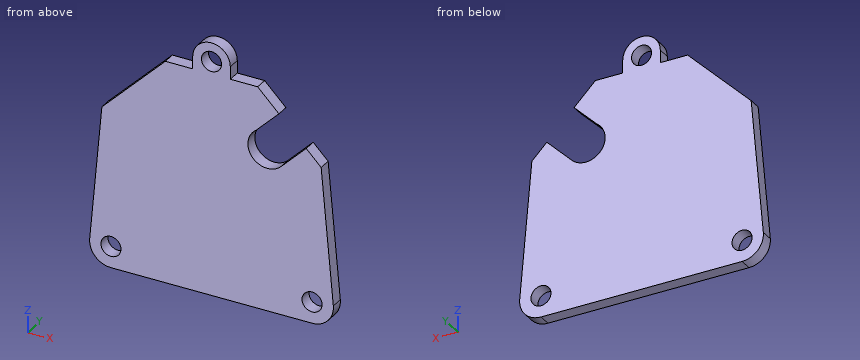
```python
from build123d import *

# Parameters (mm, degrees)
SKETCH1_R           = 1.6
BOSS_EXTRUDE1_DEPTH = 2


with BuildPart() as part:
    # Sketch1 → Boss-Extrude1 (new body)
    with BuildSketch(Plane(origin=(0, 0, 0), x_dir=(1, 0, 0), z_dir=(0, 1, 0))):
        with BuildLine():
            ThreePointArc((7.536585866, 10.5201286), (2.958706846, 10.319962474), (3.565513998, 5.778065527))
            Line((3.565513998, 5.778065527), (7.192643667, 2.150935858))
            Line((7.192643667, 2.150935858), (3.793373086, -1.248334723))
            Line((3.793373086, -1.248334723), (-0.570702654, -1.248334723))
            Line((-0.570702654, -1.248334723), (-0.570702654, -3.253047476))
            ThreePointArc((-0.570702654, -3.253047476), (-3.570702654, -6.253047476), (-6.570702654, -3.253047476))
            Line((-6.570702654, -3.253047476), (-6.570702654, -1.248334723))
            Line((-6.570702654, -1.248334723), (-10.934778393, -1.248334723))
            Line((-10.934778393, -1.248334723), (-21.070702654, 8.887589537))
            Line((-21.070702654, 8.887589537), (-23.015874855, 30.595563989))
            ThreePointArc((-23.015874855, 30.595563989), (-22.136333563, 33.200086558), (-19.620702654, 34.308568326))
            Line((-19.620702654, 34.308568326), (12.479297346, 34.308568326))
            ThreePointArc((12.479297346, 34.308568326), (14.994928256, 33.200086558), (15.874469548, 30.595563989))
            Line((15.874469548, 30.595563989), (13.929297346, 8.887589537))
            Line((13.929297346, 8.887589537), (11.545749837, 6.504042028))
            Line((11.545749837, 6.504042028), (7.536585866, 10.5201286))
        make_face()
        with Locations((-19.620702654, 30.899792953)):
            Circle(SKETCH1_R, mode=Mode.SUBTRACT)
        with Locations((12.479297346, 30.899792953)):
            Circle(SKETCH1_R, mode=Mode.SUBTRACT)
        with Locations((-3.570702654, -3.253047476)):
            Circle(SKETCH1_R, mode=Mode.SUBTRACT)
    extrude(amount=BOSS_EXTRUDE1_DEPTH)


solid = part.part
```
The model under review builds one solid part; all positions refer to its coordinate system, in mm. Round coordinates to 2 decimals unless told otherwise and drop trailing zeros. Order: outer loops, then holes, each group sorted by start corner. A loop starts at its lowest first (then second) coordinate and runs counter-clockwise, first axis right, second up. Notation, with made-up numbers: M 77,-27 L 117,-27 A10 ccw 117,-11 Z; hole C 13,-8 d3. An arc over 180 degrees is marked long. Use a Markdown table: item, result.
1) Insertion check: pin 1 (0.6 mm diameter, centred on y = 0.5, z = 2, fed in from +X); pin 2 (1 mm diameter, centred on x = -9, y = 1, fed in from +Z). Each pin has a flat end and moves straight along its axis. Give the tip position at first contact, or say it passes through.
Report:
| item | result |
|---|---|
| pin 1 | x = -0.57 |
| pin 2 | z = 1.25 |
2) Consider section C-C (x = 0). Write out the cut boundary in (y, z), then the cut area to 3 significant figures.
Report:
| item | result |
|---|---|
| outline | M 0,-34.31 L 2,-34.31 L 2,1.25 L 0,1.25 Z |
| area | 71.1 mm^2 |
3) Consider section D-D (z = -17). Write out the cut boundary in (x, y).
Report:
| item | result |
|---|---|
| outline | M -21.8,0 L 14.66,0 L 14.66,2 L -21.8,2 Z |
4) Wall thickness on line 1 along X through (y, z) = (1.55, -32); line 2 along Z through (x, y) = (-7.5, 0.65); line 3 along X through (y, z) = (0.5, -30): over which ranges is each line inside the solid? List them lowest first. Write a range as [from, to].
Report:
| item | result |
|---|---|
| line 1 | [-22.85, -20.78], [-18.46, 11.32], [13.64, 15.71] |
| line 2 | [-34.31, 1.25] |
| line 3 | [-22.96, -20.94], [-18.3, 11.16], [13.8, 15.82] |
5) Consider section B-B (y = 0.3). Write out the cut boundary in (x, z).
Report:
| item | result |
|---|---|
| outline | M -23.02,-30.6 A3.41 ccw -19.62,-34.31 L 12.48,-34.31 A3.41 ccw 15.87,-30.6 L 13.93,-8.89 L 11.55,-6.5 L 7.54,-10.52 A3.1 cw long 3.57,-5.78 L 7.19,-2.15 L 3.79,1.25 L -0.57,1.25 L -0.57,3.25 A3 ccw -6.57,3.25 L -6.57,1.25 L -10.93,1.25 L -21.07,-8.89 Z; hole C -19.62,-30.9 d3.2; hole C -3.57,3.25 d3.2; hole C 12.48,-30.9 d3.2 |
6) Consider section A-A (x = 5). Write out the cut boundary in (y, z).
Report:
| item | result |
|---|---|
| outline | M 0,-34.31 L 2,-34.31 L 2,-11.41 L 0,-11.41 Z; M 0,-4.34 L 2,-4.34 L 2,0.04 L 0,0.04 Z |
